Read the model definition and answer for the solid it produces. Units are mm, in the model's axes. A direction names the side the tool comes from. Give positions to 0.01 mm unless a question says otherwise; leave off trailing zeros. Order: outer loops, then holes, each group sorted by start corner. A loop starts at its lowest first (then second) coordinate and runs counter-clockwise, first axis right, second up. Notation, with made-up numbers: M 63.5,-32 L 99.5,-32 A19 cw 99.5,-8 Z; hole C 30,85.25 d11. An arc over 180 degrees is marked long. One line per item, written item: value.
Autodesk Inventor part; units mm, degrees
ref_plane "YZ Plane" through (0, 0, 0) normal (1, 0, 0) x (0, 1, 0)
ref_plane "XZ Plane" through (0, 0, 0) normal (0, 1, 0) x (-1, 0, 0)
ref_plane "XY Plane" through (0, 0, 0) normal (0, 0, 1) x (1, 0, 0)
sketch "Эскиз1" plane through (0, 0, 0) normal (0, 1, 0) x (-1, 0, 0)
  line L0 (0, 18) -> (0, -18)
  arc A0 (-57.1363, 7.7095) -> (-57.1363, -7.7095) centre (-55, 0) ccw
  line L1 (0, 0) -> (-6.25, 0) construction
  line L2 (0, 18) -> (-18.6401, 18)
  line L3 (-21.3105, 17.6369) -> (-57.1363, 7.7095)
  line L4 (0, -18) -> (-18.6401, -18)
  line L5 (-21.3105, -17.6369) -> (-57.1363, -7.7095)
  circle A1 centre (-55, 0) radius 2
  arc A2 (-18.6401, 18) -> (-21.3105, 17.6369) centre (-18.6401, 8) ccw
  arc A3 (-21.3105, -17.6369) -> (-18.6401, -18) centre (-18.6401, -8) ccw
  circle A4 centre (-10, -13) radius 1.75
  circle A5 centre (-10, 13) radius 1.75
  line L6 (-10, 13) -> (-10, -13) construction
  point P0 (-20, 18)
  dimension "d0" = 16
  dimension "d1" = 36
  dimension "d2" = 55
  dimension "d3" = 20
  dimension "d4" = 4
  dimension "d5" = 10
  dimension "d18" = 3.5
  dimension "d19" = 13
  dimension "d20" = 10
extrude "Выдавливание1" add sketch "Эскиз1" along normal blind 4
sketch "Эскиз2" plane through (0, 4, 0) normal (0, 1, 0) x (1, 0, 0)
  line L0 (0, 0) -> (14.985, 0) construction
  line L1 (0, 7.5) -> (22, 7.5)
  line L2 (22, 7.5) -> (22, -7.5)
  line L3 (22, -7.5) -> (0, -7.5)
  line L4 (0, -7.5) -> (0, 7.5)
  line L5 (0, 18) -> (0, -18)
  dimension "d8" = 15
  dimension "d9" = 22
extrude "Выдавливание2" add sketch "Эскиз2" along normal blind 2
chamfer "Фаска1" distance 2 angle 45 1 edges at (22, 6, 0)
chamfer "Фаска2" distance 0.5 angle 45 2 edges at (10.0002, 6, 7.5) (10.0003, 6, -7.5)
sketch "Эскиз4" plane through (0, 4, 0) normal (0, 1, 0) x (1, 0, 0)
  circle A0 centre (55, 0) radius 2
  circle A1 centre (55, 0) radius 3
  point P0 (0, 0)
  dimension "d21" = 1
extrude "Выдавливание3" add sketch "Эскиз4" along normal blind 1
chamfer "Фаска3" distance 1 angle 45 1 edges at (52, 4, 0)
properties part number "04-06-Рычаг верхний"
1) Which of the six approach directions +Z, -Z, +X, -X, +Y, -Y give full straight-line access (tool end or side, diameter ignored) to faces 1 (the face through (32, 4, 0)), 2 (the face through (57, 5, 1)), 3 (the face through (9, 2, 18)), 4 (the face through (21, 5, 0))?
Reported:
face 1: +Y
face 2: +Z, -Z, +X, +Y
face 3: +Z, +X, -X, +Y, -Y
face 4: +Z, -Z, +Y
2) Find section D-D, the plane z = -13. Write down the section's boundary in (x, y), plus the area to 3 significant figures.
Reported:
outline: M 0,0 L 8.25,0 L 8.25,4 L 0,4 Z; M 11.75,0 L 38.04,0 L 38.04,4 L 11.75,4 Z
area: 138 mm^2
3) Determine the mould class of faces 5 (the face through (10.228, 1.972, 11.265)), 6 (the face through (0, 2, 0)), 7 (the face through (11, 5, -7.5)), 8 (the face through (38.973, 1.972, -12.743)) for opening direction X: +X half, -X half, draft (parallel to the pull), parting line (faces both ways), or undercut.
Reported:
face 5: undercut
face 6: -X half
face 7: draft
face 8: +X half
4) Consider probe 1 along Z at (x, y) = (10, 2.25); probe 2 along X at (y, z) = (3.7, 0); probe 3 along Z at (x, y) = (11.5, 1.5). Determine where each line is inside the solid, lowest interval first.
Reported:
probe 1: z = -18 to -14.75, -11.25 to 11.25, 14.75 to 18
probe 2: x = 0 to 53, 57 to 63
probe 3: z = -18 to -13.9, -12.1 to 12.1, 13.9 to 18
5) Find section A-A, the plane x = 10. Write down the section's boundary in (y, z).
Reported:
outline: M 0,-18 L 4,-18 L 4,-14.75 L 0,-14.75 Z; M 0,-11.25 L 4,-11.25 L 4,-7.5 L 5.5,-7.5 L 6,-7 L 6,7 L 5.5,7.5 L 4,7.5 L 4,11.25 L 0,11.25 Z; M 0,14.75 L 4,14.75 L 4,18 L 0,18 Z
6) Each of these flat-tipped pins is pushed along its axis until it touches: pin 1 Ø3 at (x, z) = (43, -11.5) entering from +Y; pin 2 Ø6 at (x, z) = (22.5, 0) entering from +Y; pin 3 Ø5 at (x, z) = (55, 0) entering from +Y. Where does it stop, or does it pass through?
Reported:
pin 1: stops at y = 4
pin 2: stops at y = 6
pin 3: stops at y = 5
